Autodesk Inventor part; units mm, degrees
ref_plane "YZ Plane" through (0, 0, 0) normal (1, 0, 0) x (0, 1, 0)
ref_plane "XZ Plane" through (0, 0, 0) normal (0, 1, 0) x (-1, 0, 0)
ref_plane "XY Plane" through (0, 0, 0) normal (0, 0, 1) x (1, 0, 0)
sketch "Sketch1" plane through (0, 0, 0) normal (0, 0, 1) x (1, 0, 0)
  line L0 (204.17, 231.1255) -> (241.5918, 231.1255)
  line L1 (241.5918, 231.1255) -> (284.0136, 231.1255)
  line L2 (204.17, 226.1255) -> (241.5918, 226.1255)
  line L3 (246.5918, 226.1255) -> (284.0136, 226.1255)
  line L4 (246.5918, 188.7037) -> (246.5918, 226.1255)
  line L5 (246.5918, 231.1255) -> (246.5918, 268.5473)
  line L6 (241.5918, 188.7037) -> (241.5918, 226.1255)
  line L7 (241.5918, 231.1255) -> (241.5918, 268.5473)
  line L8 (241.5918, 231.1255) -> (288.8318, 231.1255) construction
  line L9 (246.5918, 231.1255) -> (303.9178, 231.1255) construction
  line L10 (246.5918, 288.5734) -> (304.1186, 288.5734) construction
  circle A0 centre (244.0918, 228.6255) radius 40
  line L11 (246.5918, 226.1255) -> (249.8364, 189.0401)
  line L12 (246.5918, 226.1255) -> (283.8188, 226.1255) construction
  line L13 (283.8188, 226.1255) -> (246.5918, 222.8685)
  line L14 (283.8188, 226.1255) -> (321.1881, 226.1255) construction
  line L15 (246.5918, 231.1255) -> (283.6772, 234.37)
  line L16 (246.5918, 268.3525) -> (249.8488, 231.1255)
  line L17 (241.5918, 231.1255) -> (238.3473, 268.2108)
  line L18 (204.3648, 231.1255) -> (241.5918, 234.3824)
  line L19 (241.5918, 226.1255) -> (204.5065, 222.8809)
  line L20 (241.5918, 188.8985) -> (238.3349, 226.1255)
  point P0 (0, 0)
  point P1 (303.8392, 234.1257)
  point P2 (241.3091, 234.3577)
  point P3 (249.824, 231.4082)
  point P4 (238.3596, 225.8427)
  point P5 (246.8746, 222.8933)
  dimension "d31" = 80
  dimension "d33" = 85
  dimension "d34" = 175
  dimension "d37" = 360
extrude "Extrusion1" add sketch "Sketch1" along normal blind 45
extrude "Extrusion2" cut sketch "Sketch1" along normal blind 40 contours A0 L17 L18 L0 | L19 L20 L6 A0 | A0 L15 L16 L5 | L11 L13 L3 A0
extrude "Extrusion4" add sketch "Sketch1" along normal blind 5 contours A0 L17 L18 L0 | L19 L20 L6 A0 | A0 L15 L16 L5 | L11 L13 L3 A0
ref_plane "Work Plane1" through (244.0918, 228.6255, 0) normal (0, 0, -1) x (-1, 0, 0)
sketch "Sketch2" plane through (244.0918, 228.6255, 0) normal (0, 0, -1) x (-1, 0, 0)
  circle A0 centre (0, 0) radius 4
  point P0 (244.0918, -228.6255)
  dimension "d28" = 8
extrude "Extrusion5" cut sketch "Sketch2" against normal blind 10
properties part number "wheel"
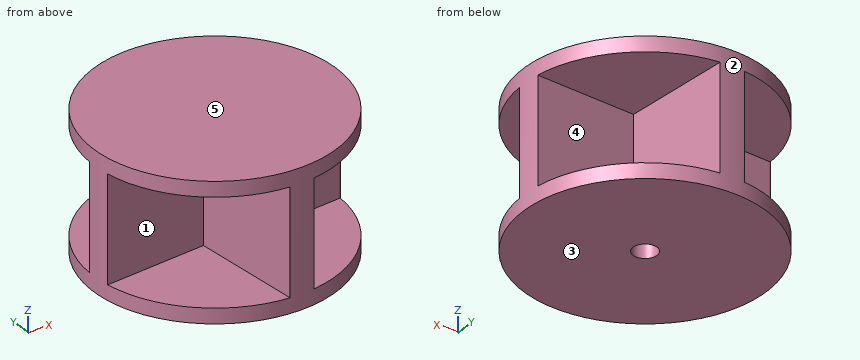
Check sheet for the modelled part. Datum: model origin and axes. Units: mm. Face numbers are marked on the shaded views. A direction names the side the tool comes from. Coordinates: 2 decimals unless noted, no trailing zeros. Order: outer loops, then holes, each group sorted by start corner. A loop starts at its lowest first (then second) coordinate and runs counter-clockwise, first axis right, second up. Notation, with made-up numbers: M 76.5,-12.5 L 118.5,-12.5 A33 ccw 118.5,24.5 Z; hole C 9,-27.75 d2. An arc over 180 degrees is marked long. One line per question, with ' | ' between items. Start each with the question number.
Item 1: Material ranges on line 1 (Z direction, x = 250, y = 257.5); line 2 (X direction, y = 228.5, z = 9); line 3 (Y direction, x = 243.5, z = 27.5), recorded low to high.
Item 2: Sectioned sample at B-B on x = 262.5. Record the cut outline in (y, z), and give its area (3 significant figures).
Item 3: Sectioned sample at D-D on z = 42.5. Record the cut outline in (x, y), and give its area (3 significant figures).
Item 4: Gauge pin test, flat ends, axial feed: P1, Ø1.5, axis at x = 264.5, z = 7, coming from the -Y side; P2, Ø5, axis at x = 257.5, z = 30, coming from the -Y side; P3, Ø1.5, axis at y = 236.5, z = 24, coming from the +X side. Record the tip position at first contact, or that the pin passes through.
Item 5: Sectioned sample at A-A on z = 18. Record the cut outline in (x, y).
Item 6: Sectioned sample at C-C on y = 248. Record the cut outline in (x, z), and give its area (3 significant figures).
Item 7: Access from +Z, -Z, +X, -X, +Y, -Y to the whole of each face (thin tool, end or side, straight path). Record for the marked faces 1 and 2.
Item 8: Mould release check, pull along Z, two halves, no side actions. Record for the marked faces 3, 4 and 5: pulls with the +Z half, pulls with the -Z half, needs draft (parallel to the pull), parting line crosses it, or undercut.
Answer below:
1) line 1: z = 0 to 5, 40 to 45 | line 2: x = 204.09 to 240.09, 248.09 to 284.09 | line 3: y = 188.63 to 268.62
2) outline: M 193.11,0 L 264.14,0 L 264.14,5 L 232.52,5 L 232.52,40 L 264.14,40 L 264.14,45 L 193.11,45 L 193.11,40 L 224.26,40 L 224.26,5 L 193.11,5 Z | area: 999 mm^2
3) outline: C 244.09,228.63 d80 | area: 5,030 mm^2
4) P1: stops at y = 224.37 | P2: stops at y = 223.6 | P3: stops at x = 249.44
5) outline: M 204.17,231.13 A40 ccw 204.51,222.88 L 238.36,225.84 L 241.59,188.9 L 241.59,188.7 A40 ccw 249.84,189.04 L 246.87,222.89 L 283.82,226.13 L 284.01,226.13 A40 ccw 283.68,234.37 L 249.82,231.41 L 246.59,268.35 L 246.59,268.55 A40 ccw 238.35,268.21 L 241.31,234.36 L 204.36,231.13 Z
6) outline: M 209.1,0 L 279.09,0 L 279.09,5 L 248.37,5 L 248.37,40 L 279.09,40 L 279.09,45 L 209.1,45 L 209.1,40 L 240.12,40 L 240.12,5 L 209.1,5 Z | area: 989 mm^2
7) face 1: -Y | face 2: +Z, -Z
8) face 3: pulls with the -Z half | face 4: undercut | face 5: pulls with the +Z half
